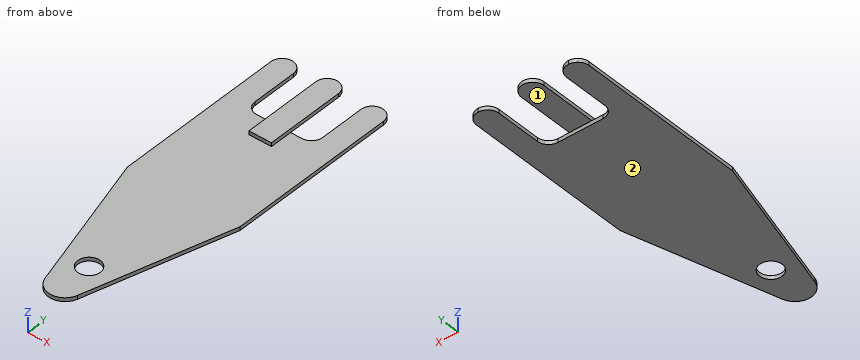
from build123d import *

# Parameters (mm, degrees)
F1_DEPTH    = 1.05
F2_R        = 3.175
F3_DEPTH    = 28.1652770936
F4_T1_DEPTH = 16.925
F6_DEPTH    = 1.05
F7_DEPTH    = 6.35
F8_DEPTH    = 1.05
F9_R        = 3.175


# Not quite as in the source:
# - a fillet or chamfer that OpenCascade refuses, or shapes differently, is made with other operations: its cross-section is extruded or revolved along the edge and cut away or added


with BuildPart() as f1:
    # F0 (on Top) → F1 (new body)
    with BuildSketch(Plane.XY):
        Polygon((-15.875, 0), (15.875, 0), (15.875, 50.8), (9.525, 50.8), (9.525, 31.75), (3.175, 31.75), (3.175, 50.8), (-3.175, 50.8), (-3.175, 31.75), (-9.525, 31.75), (-9.525, 50.8), (-15.875, 50.8), align=None)
        with BuildLine():
            Line((4.5889374784, -40.6525160217), (15.875, 0))
            Line((15.875, 0), (-15.875, 0))
            Line((-15.875, 0), (-4.5889374784, -40.6525160217))
            ThreePointArc((-4.5889374784, -40.6525160217), (0, -44.1410226664), (4.5889374784, -40.6525160217))
        make_face()
    extrude(amount=F1_DEPTH)

    # F2 (on face) → F3 (cut)
    with BuildSketch(Plane.XY):
        with Locations((0, -31.4410226664)):
            Circle(F2_R)
    extrude(amount=F3_DEPTH, mode=Mode.SUBTRACT)

    # F4: fillet of radius 3.175 on 6 edges, made by hand

    # F4_s2 → F4_t1 (cut)
    with BuildSketch(Plane.XY.offset(-7.9375)):
        with BuildLine():
            ThreePointArc((15.875, 47.625), (14.9450640303, 49.8700640303), (12.7, 50.8))
            Line((12.7, 50.8), (15.875, 50.8))
            Line((15.875, 50.8), (15.875, 47.625))
        make_face()
        with BuildLine():
            ThreePointArc((12.7, 50.8), (10.4549359697, 49.8700640303), (9.525, 47.625))
            Line((9.525, 47.625), (9.525, 50.8))
            Line((9.525, 50.8), (12.7, 50.8))
        make_face()
        with BuildLine():
            ThreePointArc((3.175, 47.625), (2.2450640303, 49.8700640303), (0, 50.8))
            Line((0, 50.8), (3.175, 50.8))
            Line((3.175, 50.8), (3.175, 47.625))
        make_face()
        with BuildLine():
            ThreePointArc((0, 50.8), (-2.2450640303, 49.8700640303), (-3.175, 47.625))
            Line((-3.175, 47.625), (-3.175, 50.8))
            Line((-3.175, 50.8), (0, 50.8))
        make_face()
        with BuildLine():
            ThreePointArc((-12.7, 50.8), (-10.4549359697, 49.8700640303), (-9.525, 47.625))
            Line((-9.525, 47.625), (-9.525, 50.8))
            Line((-9.525, 50.8), (-12.7, 50.8))
        make_face()
        with BuildLine():
            ThreePointArc((-15.875, 47.625), (-14.9450640303, 49.8700640303), (-12.7, 50.8))
            Line((-12.7, 50.8), (-15.875, 50.8))
            Line((-15.875, 50.8), (-15.875, 47.625))
        make_face()
    extrude(amount=F4_T1_DEPTH, mode=Mode.SUBTRACT)

    # F5 (on face) → F6 (join)
    with BuildSketch(Plane.XY.offset(1.05)):
        with BuildLine():
            Line((-3.175, 47.625), (-3.175, 31.75))
            Line((-3.175, 31.75), (3.175, 31.75))
            Line((3.175, 31.75), (3.175, 47.625))
            ThreePointArc((3.175, 47.625), (0, 50.8), (-3.175, 47.625))
        make_face()
    extrude(amount=F6_DEPTH)

    # F7 (add): a face of the model
    f7_faces = [f1.faces().sort_by_distance(p)[0] for p in [
        (0, 31.75, 1.575),
    ]]
    extrude(f7_faces, amount=F7_DEPTH)

    # F5 (on face) → F8 (cut)
    with BuildSketch(Plane.XY.offset(1.05)):
        with BuildLine():
            Line((-3.175, 47.625), (-3.175, 31.75))
            Line((-3.175, 31.75), (3.175, 31.75))
            Line((3.175, 31.75), (3.175, 47.625))
            ThreePointArc((3.175, 47.625), (0, 50.8), (-3.175, 47.625))
        make_face()
    extrude(amount=-F8_DEPTH, mode=Mode.SUBTRACT)

    # F9
    f9_edges = [f1.edges().sort_by_distance(p)[0] for p in [
        (-9.525, 31.75, 0.525),
        (9.525, 31.75, 0.525),
    ]]
    fillet(f9_edges, radius=F9_R)


solid = f1.part
Geometry check sheet. Reference: the model listing, model coordinates, mm. Face numbers are marked on the shaded views. A direction names the side the tool comes from. Round coordinates to 2 decimals unless told otherwise and drop trailing zeros. Order: outer loops, then holes, each group sorted by start corner. A loop starts at its lowest first (then second) coordinate and runs counter-clockwise, first axis right, second up. Notation, with made-up numbers: M 4,5 L 52,5 A20 ccw 52,18 Z; hole C -3,14.5 d11. An arc over 180 degrees is marked long. Answer in a Markdown table with one row per item. Add a question column.
Item 1: Material ranges on L1, parallel to X at y = 46.5, z = 0.7 (3 decimals); L2, parallel to Y at x = 0, z = 0.25, recorded low to high. Write a range as [from, to].
Item 2: Set-up check for the marked faces 1 and 2: record each of +Z, -Z, +X, -X, +Y, -Y from which the full face is reachable in a straight line by a thin tool's end or side.
Item 3: Sectioned sample at A-A, the plane x = 0. Enter the section's corners in (y, z), plus the area to 3 significant figures.
Item 4: Sectioned sample at C-C, the plane y = -24.5. Enter the section's corners in (x, z).
Item 5: Depth check by flat-ended pin: pin 1 Ø1.9 at (x, y) = (-1.5, 37.5) entering from -Z; pin 2 Ø0.5 at (x, z) = (-2.5, 0.5) entering from +Y; pin 3 Ø4 at (x, y) = (10.5, 32) entering from +Z; pin 4 Ø3 at (x, y) = (-12, 4.5) entering from -Z. Enter the tip coordinate at first touch or a pass-through.
Item 6: Sectioned sample at D-D, the plane x = -11. Enter the section's corners in (y, z), plus the area to 3 significant figures.
Filled in:
| question | item | result |
|---|---|---|
| 1 | L1 | x = [-15.875, -9.525], [9.525, 15.875] |
| 1 | L2 | y = [-44.14, -34.62], [-28.27, 31.75] |
| 2 | face 1 | -Z, +Y |
| 2 | face 2 | -Z, +X, -X, +Y, -Y |
| 3 | outline | M -44.14,0 L -34.62,0 L -34.62,1.05 L -44.14,1.05 Z; M -28.27,0 L 31.75,0 L 31.75,1.05 L 50.8,1.05 L 50.8,2.1 L 25.4,2.1 L 25.4,1.05 L -28.27,1.05 Z |
| 3 | area | 99.7 mm² |
| 4 | outline | M -9.07,0 L 9.07,0 L 9.07,1.05 L -9.07,1.05 Z |
| 5 | pin 1 | stops at z = 1.05 |
| 5 | pin 2 | stops at y = 31.75 |
| 5 | pin 3 | stops at z = 1.05 |
| 5 | pin 4 | stops at z = 0 |
| 6 | outline | M -17.56,0 L 50.31,0 L 50.31,1.05 L -17.56,1.05 Z |
| 6 | area | 71.3 mm² |
